```python
from build123d import *
from build123d.topology import SkipClean

# Parameters (mm, degrees)
BOSS_EXTRUDE2_DEPTH = 3.175
SKETCH3_R           = 9.700000031
BOSS_EXTRUDE4_DEPTH = 3.175
SKETCH4_R           = 1.0033
CUT_EXTRUDE1_DEPTH  = 3.175
SKETCH6_R           = 1.25
CUT_EXTRUDE2_DEPTH  = 18.630160878
CUT_EXTRUDE3_DEPTH  = 18.630161045
CUT_EXTRUDE4_DEPTH  = 18.630161045
SKETCH9_R           = 3.2385
CUT_EXTRUDE5_DEPTH  = 18.630161045
SKETCH11_R          = 1.377
CUT_EXTRUDE7_DEPTH  = 18.630161045


with BuildPart() as part:
    # Sketch1 → Boss-Extrude2 (new body)
    with BuildSketch(Plane(origin=(0, 0, 0), x_dir=(1, 0, 0), z_dir=(0, 1, 0))):
        with BuildLine():
            ThreePointArc((-11.359521952, 7.075729248), (-11.584059991, 5.734660127), (-10.793437735, 4.628405109))
            Line((-10.793437735, 4.628405109), (-9.903263338, 4.073924644))
            ThreePointArc((-9.903263338, 4.073924644), (-9.442762789, 3.620550105), (-9.219865441, 3.013981065))
            ThreePointArc((-9.219865441, 3.013981065), (-8.233383025, 5.128489502), (-6.770495536, 6.946250125))
            ThreePointArc((-6.770495536, 6.946250125), (-7.413198477, 6.878854591), (-8.023169667, 7.092265875))
            Line((-8.023169667, 7.092265875), (-8.913344063, 7.64674634))
            ThreePointArc((-8.913344063, 7.64674634), (-10.254863148, 7.868580207), (-11.359521952, 7.075729248))
        make_face()
        with BuildLine():
            ThreePointArc((-7.092265875, -8.023169667), (-6.878854591, -7.413198477), (-6.946250125, -6.770495536))
            ThreePointArc((-6.946250125, -6.770495536), (5.128489502, 8.233383025), (-3.013981065, -9.219865441))
            ThreePointArc((-3.013981065, -9.219865441), (-3.620550105, -9.442762789), (-4.073924644, -9.903263338))
            Line((-4.073924644, -9.903263338), (-4.628405109, -10.793437735))
            ThreePointArc((-4.628405109, -10.793437735), (-5.734660127, -11.584059991), (-7.075729248, -11.359521952))
            ThreePointArc((-7.075729248, -11.359521952), (-7.868580207, -10.254863148), (-7.64674634, -8.913344063))
            Line((-7.64674634, -8.913344063), (-7.092265875, -8.023169667))
        make_face()
        with BuildLine():
            ThreePointArc((4.073924644, 9.903263338), (3.620550105, 9.442762789), (3.013981065, 9.219865441))
            ThreePointArc((3.013981065, 9.219865441), (5.128489502, 8.233383025), (6.946250125, 6.770495536))
            ThreePointArc((6.946250125, 6.770495536), (6.878854591, 7.413198477), (7.092265875, 8.023169667))
            Line((7.092265875, 8.023169667), (7.64674634, 8.913344063))
            ThreePointArc((7.64674634, 8.913344063), (7.868580207, 10.254863148), (7.075729248, 11.359521952))
            ThreePointArc((7.075729248, 11.359521952), (5.734660127, 11.584059991), (4.628405109, 10.793437735))
            Line((4.628405109, 10.793437735), (4.073924644, 9.903263338))
        make_face()
        with BuildLine():
            ThreePointArc((9.903263338, -4.073924644), (9.442762789, -3.620550105), (9.219865441, -3.013981065))
            ThreePointArc((9.219865441, -3.013981065), (8.233383025, -5.128489502), (6.770495536, -6.946250125))
            ThreePointArc((6.770495536, -6.946250125), (7.413198477, -6.878854591), (8.023169667, -7.092265875))
            Line((8.023169667, -7.092265875), (8.913344063, -7.64674634))
            ThreePointArc((8.913344063, -7.64674634), (10.254863148, -7.868580207), (11.359521952, -7.075729248))
            ThreePointArc((11.359521952, -7.075729248), (11.584059991, -5.734660127), (10.793437735, -4.628405109))
            Line((10.793437735, -4.628405109), (9.903263338, -4.073924644))
        make_face()
    extrude(amount=BOSS_EXTRUDE2_DEPTH)

    # Sketch3 → Boss-Extrude4 (add)
    with BuildSketch(Plane(origin=(0, 3.175, 0), x_dir=(1, 0, 0), z_dir=(0, 1, 0))):
        with Locations(Location((0, 0, 0), (0, 0, 71.897391919))):
            Circle(SKETCH3_R)
    extrude(amount=BOSS_EXTRUDE4_DEPTH)

    # Sketch4 → Cut-Extrude1 (cut)
    with BuildSketch(Plane(origin=(0, 3.175, 0), x_dir=(1, 0, 0), z_dir=(0, 1, 0))):
        with Locations(Location((-6.102109375, -9.796452489, 0), (0, 0, 270))):
            Circle(SKETCH4_R)
        with Locations(Location((-9.796452489, 6.102109375, 0), (0, 0, 270))):
            Circle(SKETCH4_R)
        with Locations(Location((6.102109375, 9.796452489, 0), (0, 0, 270))):
            Circle(SKETCH4_R)
        with Locations(Location((9.796452489, -6.102109375, 0), (0, 0, 270))):
            Circle(SKETCH4_R)
    extrude(amount=-CUT_EXTRUDE1_DEPTH, mode=Mode.SUBTRACT)

    # Sketch6 → Cut-Extrude2 (cut, through all)
    with BuildSketch(Plane.XZ):
        with Locations(Location((-4.120304599, 6.857338406, 0), (0, 0, 270))):
            Circle(SKETCH6_R)
        with Locations(Location((6.857338406, 4.120304599, 0), (0, 0, 270))):
            Circle(SKETCH6_R)
        with Locations(Location((4.120304599, -6.857338406, 0), (0, 0, 270))):
            Circle(SKETCH6_R)
        with Locations(Location((-6.857338406, -4.120304599, 0), (0, 0, 270))):
            Circle(SKETCH6_R)
        with BuildLine():
            ThreePointArc((-7.740826737, 4.188918313), (-8.600917053, 2.001520862), (-8.865312738, -0.333978632))
            ThreePointArc((-8.865312738, -0.333978632), (-8.220855367, -1.436176951), (-6.960889199, -1.642699812))
            add(Edge.make_bspline(
                [(-6.960889199, -1.642699812), (-6.667021958, -1.55913113), (-6.387287356, -1.541557431)],
                knots=[0, 0, 0, 1, 1, 1], degree=2))
            ThreePointArc((-6.387287356, -1.541557431), (-5.348606232, -1.027965094), (-4.985782131, 0.07248674))
            ThreePointArc((-4.985782131, 0.07248674), (-4.766455839, 1.294643053), (-4.258288499, 2.427575545))
            ThreePointArc((-4.258288499, 2.427575545), (-4.213628063, 3.537788389), (-4.945115585, 4.374145441))
            add(Edge.make_bspline(
                [(-4.945115585, 4.374145441), (-5.082112842, 4.444222059), (-5.247145609, 4.565325221), (-5.339984058, 4.633451266), (-5.43868295, 4.713583878)],
                knots=[0, 0, 0, 0.6, 0.6, 1, 1, 1], degree=2))
            ThreePointArc((-5.43868295, 4.713583878), (-6.717452114, 5.011565124), (-7.740826737, 4.188918313))
        make_face()
    extrude(amount=-CUT_EXTRUDE2_DEPTH, mode=Mode.SUBTRACT)

    # Sketch7 → Cut-Extrude3 (cut, through all)
    with SkipClean():  # the faces are left unmerged after this step: merging them gives an invalid solid
        with BuildSketch(Plane.XZ):
            with BuildLine():
                ThreePointArc((-6.960889199, -1.642699812), (-8.884242595, -1.255389349), (-9.685199878, 0.535634133))
                ThreePointArc((-9.685199878, 0.535634133), (-9.438161419, 2.238550786), (-8.894109958, 3.871021655))
                ThreePointArc((-8.894109958, 3.871021655), (-7.375413308, 5.149500563), (-5.43868295, 4.713583878))
                ThreePointArc((-5.43868295, 4.713583878), (-6.717452114, 5.011565124), (-7.740826737, 4.188918313))
                ThreePointArc((-7.740826737, 4.188918313), (-8.600917053, 2.001520862), (-8.865312738, -0.333978632))
                ThreePointArc((-8.865312738, -0.333978632), (-8.220855367, -1.436176951), (-6.960889199, -1.642699812))
            make_face()
        extrude(amount=-CUT_EXTRUDE3_DEPTH, mode=Mode.SUBTRACT)

    # Sketch8 → Cut-Extrude4 (cut, through all)
    with SkipClean():  # the faces are left unmerged after this step: merging them gives an invalid solid
        with BuildSketch(Plane.XZ):
            with BuildLine():
                Line((-9.60430299, -1.35917794), (-10.364546908, 0.869720512))
                Line((-10.364546908, 0.869720512), (-8.848022827, 0.869720512))
                Line((-8.848022827, 0.869720512), (-9.066395788, -1.091827064))
                ThreePointArc((-9.066395788, -1.091827064), (-9.431806259, -1.031432276), (-9.60430299, -1.35917794))
            make_face()
            with BuildLine():
                Line((-8.296144244, 3.19654695), (-7.610330094, 5.047226445))
                ThreePointArc((-7.610330094, 5.047226445), (-7.963941166, 5.15736977), (-7.97087416, 5.527672722))
                Line((-7.97087416, 5.527672722), (-9.651132171, 3.877614498))
                Line((-9.651132171, 3.877614498), (-8.296144244, 3.19654695))
            make_face()
        extrude(amount=-CUT_EXTRUDE4_DEPTH, mode=Mode.SUBTRACT)

    # Sketch9 → Cut-Extrude5 (cut, through all)
    with SkipClean():  # the faces are left unmerged after this step: merging them gives an invalid solid
        with BuildSketch(Plane.XZ):
            with Locations(Location((0, 0, 0), (0, 0, 270))):
                Circle(SKETCH9_R)
        extrude(amount=-CUT_EXTRUDE5_DEPTH, mode=Mode.SUBTRACT)

    # Sketch11 → Cut-Extrude7 (cut, through all)
    with SkipClean():  # the faces are left unmerged after this step: merging them gives an invalid solid
        with BuildSketch(Plane(origin=(0, 6.35, 0), x_dir=(1, 0, 0), z_dir=(0, 1, 0))):
            with Locations(Location((-6.857338406, 4.120304599, 0), (0, 0, 270))):
                Circle(SKETCH11_R)
            with Locations(Location((4.120304599, 6.857338406, 0), (0, 0, 270))):
                Circle(SKETCH11_R)
            with Locations(Location((6.857338406, -4.120304599, 0), (0, 0, 270))):
                Circle(SKETCH11_R)
            with Locations(Location((-4.120304599, -6.857338406, 0), (0, 0, 270))):
                Circle(SKETCH11_R)
        extrude(amount=-CUT_EXTRUDE7_DEPTH, mode=Mode.SUBTRACT)


solid = part.part
```
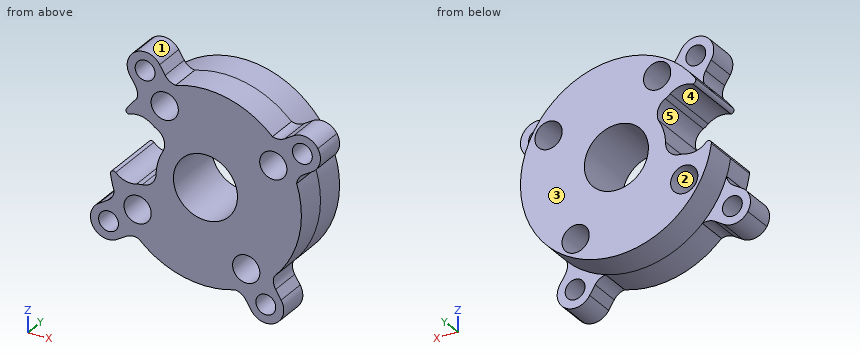
For this review, take the finished solid that the model builds, in its own axes (mm). Face numbers are marked on the shaded views. A direction names the side the tool comes from. Round coordinates to 2 decimals unless told otherwise and drop trailing zeros. Write each loop counter-clockwise with the first axis right and the second up, starting at its lowest first coordinate (ties: lowest second). Pieces come first, ordered by that corner, then holes. Notation, with made-up numbers: M 68,82.5 L 121,82.5 A22 cw 121,89.5 Z; hole C 54.25,-39 d10. An arc over 180 degrees is marked long. One line per item, written item: value. Start each with the question number.
(1) Machinability: for the marked faces 4 and 5, which of the approach directions +Z, -Z, +X, -X, +Y, -Y give a long, thin tool a straight path to every point of the face, cutting with its end or side? Answer none if there is none.
(2) Wall thickness on line 1 (X direction, y = 0.75, z = 7.75); line 2 (Z direction, x = -6.25, y = 1.25); line 3 (Z direction, x = 7, y = 3): over which ranges is each line inside the solid? List them lowest first.
(3) The part is to be moulded in two halves that separate along X. For the marked faces 1, 2 and 3, say which applies: released by +X, released by -X, zero draft, split by the parting line, or undercut.
(4) Insertion check: pin 1 (1.5 mm diameter, centred on x = -7.5, z = -0.5, fed in from -Y); pin 2 (3 mm diameter, centred on y = 2, z = -9, fed in from +X); pin 3 (3 mm diameter, centred on x = -9.8, z = -6.1, fed in from +Y) (3 decimals). Each pin has a flat end and moves straight along its axis. Give the tip position at first contact, or say it passes through.
(5) We need section B-B (z = 6.5). Give the boundary of the cut face in (x, y) (3 decimals).
(6) We need section C-C (y = 4). Count the separate pieces of the cut face and the enclosed holes in it, and give its area (3 significant figures).
Result:
1. face 4: +Y, -Y
1. face 5: -X, +Y, -Y
2. line 1: -6.96 to -5.17, -3.07 to 5.83, 9.1 to 10.6
2. line 2: -7.42 to -5.36, -2.88 to -1.53, 5.13 to 8.8, 10.79 to 11.63
2. line 3: -11.4 to -10.24, -9.35 to -7.85, -6.71 to 2.75, 5.49 to 6.89
3. face 1: split by the parting line
3. face 2: undercut
3. face 3: zero draft
4. pin 1: through
4. pin 2: x = 7.92
4. pin 3: y = 3.175
5. outline: M -7.2,0 L -5.45,0 L -5.45,6.35 L -7.2,6.35 Z; M -2.79,0 L 8.875,0 L 8.875,3.175 L 7.2,3.175 L 7.2,6.35 L -2.79,6.35 Z; M 10.717,0 L 11.592,0 L 11.592,3.175 L 10.717,3.175 Z
6. separate pieces: 1
6. enclosed holes: 5
6. area: 209 mm²
